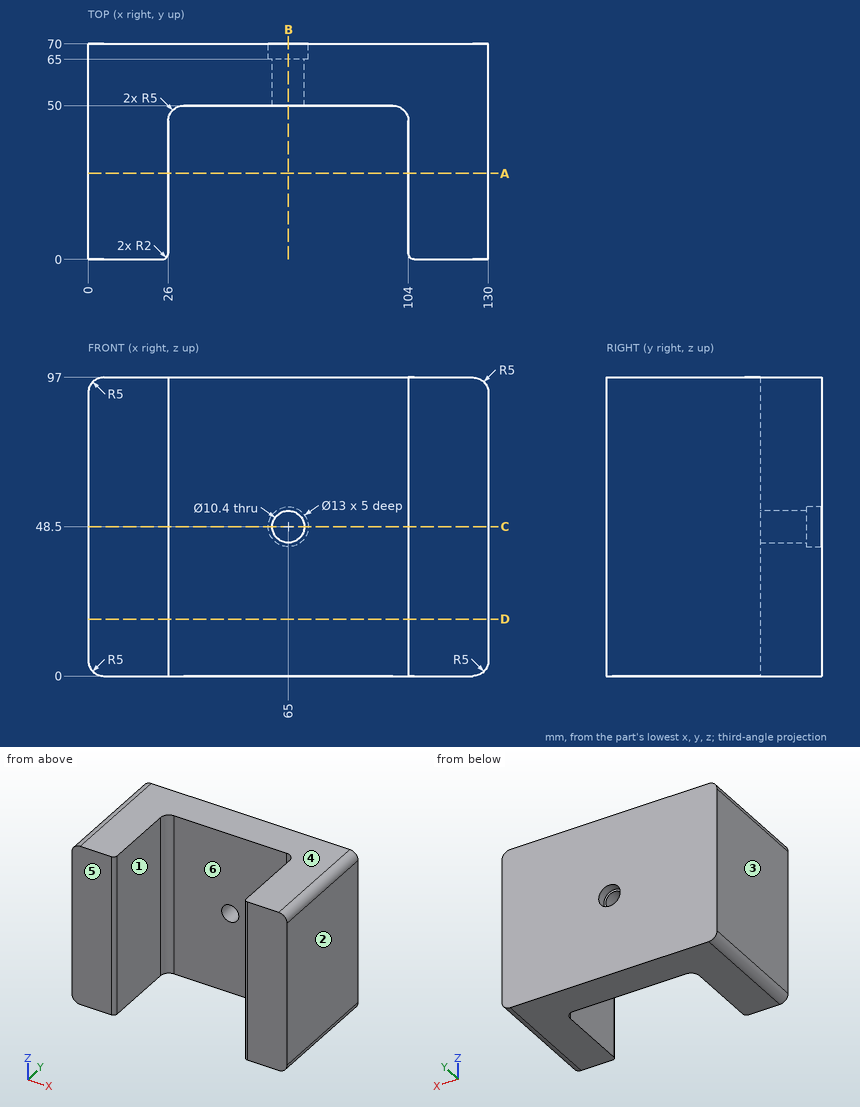
Geometry check sheet. Reference: drawing and pictorial views, mm from the part's lowest x, y, z. A direction names the side the tool comes from. Give positions to 0.01 mm unless a question says otherwise; leave off trailing zeros. Write each loop counter-clockwise with the first axis right and the second up, starting at its lowest first coordinate (ties: lowest second). Pieces come first, ordered by that corner, then holes. Notation, with made-up numbers: M 43.25,-30.75 L 83.25,-30.75 A19 ccw 83.25,-7.75 Z; hole C 52,62 d5. An arc over 180 degrees is marked long. Put each result on its own line as item: value. Start each with the question number.
1. Draft check along X on the marked faces 1, 2, 3 and 4. Enter one of: +X half, -X half, draft (parallel to the pull), parting line (faces both ways), or undercut.
2. Section check D-D (z = 18.5). Record the cut outline in (x, y), and give its area (3 significant figures).
3. Go/stop test with a flat-tipped pin: pin 1 Ø21 at (x, z) = (65, 48.5) entering from -Y. Record where the tip stops, or that it passes through.
4. Set-up check for the marked faces 5 and 6: record each of +Z, -Z, +X, -X, +Y, -Y from which the full face is reachable in a straight line by a thin tool's end or side.
5. Section check B-B (x = 65). Record the cut outline in (y, z), and give its area (3 significant figures).
6. Section check C-C (z = 48.5). Record the cut outline in (x, y), and give its area (3 significant figures).
7. Section check A-A (y = 28). Record the cut outline in (x, z).
8. Scan lines: line 1 along X through (y, z) = (38, 58.5); line 2 along X through (y, z) = (67.45, 48.5); line 3 along Y through (x, z) = (65.5, 39). Record each from-to range of solid material in increasing order. Write a range as [from, to].
Answer list:
1. face 1: undercut
1. face 2: +X half
1. face 3: -X half
1. face 4: draft
2. outline: M 0,0 L 24,0 A2 ccw 26,2 L 26,45 A5 cw 31,50 L 99,50 A5 cw 104,45 L 104,2 A2 ccw 106,0 L 130,0 L 130,70 L 0,70 Z
2. area: 5,210 mm2
3. pin 1: y = 50
4. face 5: +Z, -Z, +X, -X, -Y
4. face 6: +Z, -Z, -Y
5. outline: M 50,0 L 70,0 L 70,42 L 65,42 L 65,43.3 L 50,43.3 Z; M 50,53.7 L 65,53.7 L 65,55 L 70,55 L 70,97 L 50,97 Z
5. area: 1,720 mm2
6. outline: M 0,0 L 24,0 A2 ccw 26,2 L 26,45 A5 cw 31,50 L 59.8,50 L 59.8,65 L 58.5,65 L 58.5,70 L 0,70 Z; M 70.2,50 L 99,50 A5 cw 104,45 L 104,2 A2 ccw 106,0 L 130,0 L 130,70 L 71.5,70 L 71.5,65 L 70.2,65 Z
6. area: 4,990 mm2
7. outline: M 0,5 A5 ccw 5,0 L 26,0 L 26,97 L 5,97 A5 ccw 0,92 Z; M 104,0 L 125,0 A5 ccw 130,5 L 130,92 A5 ccw 125,97 L 104,97 Z
8. line 1: [0, 26], [104, 130]
8. line 2: [0, 58.5], [71.5, 130]
8. line 3: [50, 70]
